Here's the drawing with two shaded views (mm, measured from the low corner). I have some questions. A direction names the side the tool comes from. Coordinates: 2 decimals unless noted, no trailing zeros. Write each loop counter-clockwise with the first axis right and the second up, starting at its lowest first coordinate (ties: lowest second). Pieces come first, ordered by that corner, then holes.
Item 1: If we section it at A-A (y = 27): Please give me the cut outline in (x, z).
Item 2: I'm going to push flat-ended pins straight in: pin 1 Ø5 at (x, y) = (7.5, 9.5) entering from +Z; pin 2 Ø3 at (x, z) = (1, 4.5) entering from +Y; pin 3 Ø1 at (x, y) = (1, 32.5) entering from -Z; pin 4 Ø1 at (y, z) = (66.5, 2) entering from +X. Where does each tip first touch, or does it pass through?
Item 3: If I drill on line 1 (X direction, y = 10.5, z = 5.25); line 2 (Y direction, x = 6.75, z = 3.5), over which ranges is the centre line in solid material (lowest first)?
Item 4: For the marked faces 1 and 2, which set-ups out of +Z, -Z, +X, -X, +Y, -Y let a thin tool reach every point of the face, with its end or its side?
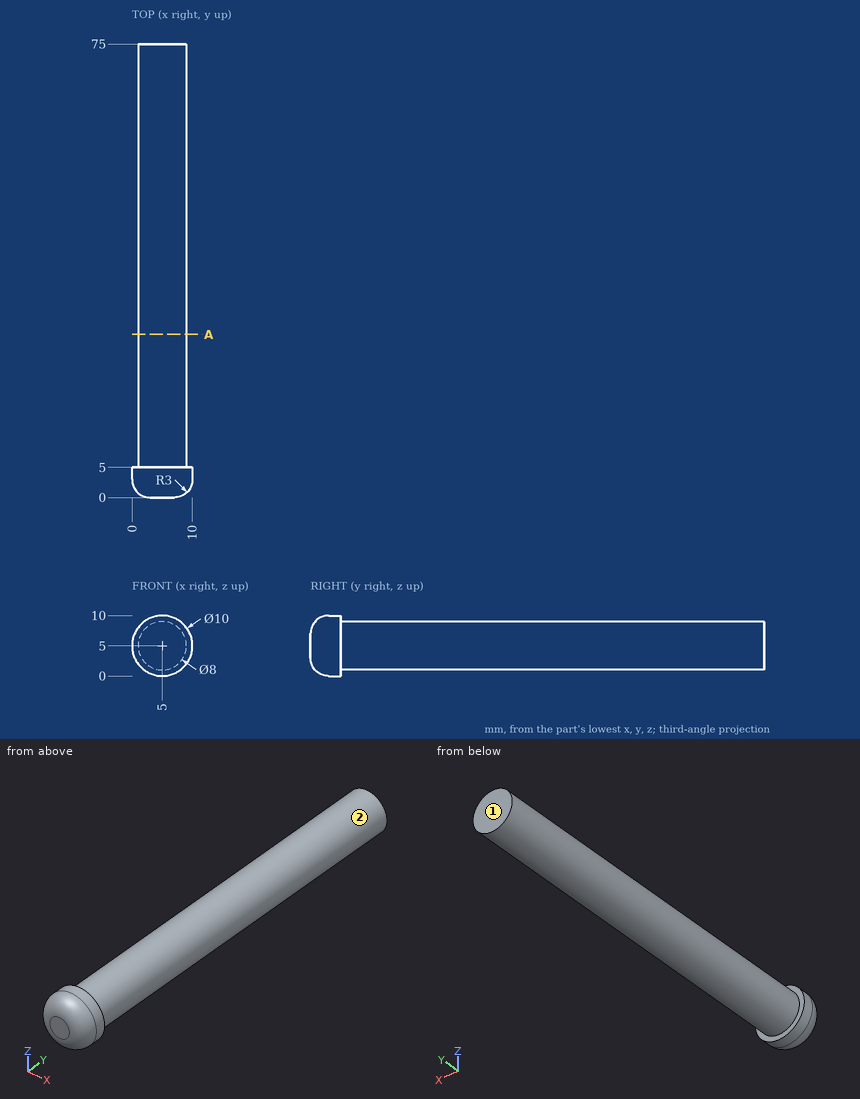
Answer list:
1. outline: circle Ø8 at (5, 5)
2. pin 1: stops at z = 9
2. pin 2: stops at y = 75
2. pin 3: stops at z = 3.06
2. pin 4: stops at x = 8.12
3. line 1: x = 1.01 to 8.99
3. line 2: y = 0.02 to 75
4. face 1: +Z, -Z, +X, -X, +Y
4. face 2: +Y
